Geometry: final body of the model. Coordinates: model frame, mm. A direction names the side the tool comes from. Round coordinates to 2 decimals unless told otherwise and drop trailing zeros. Write each loop counter-clockwise with the first axis right and the second up, starting at its lowest first coordinate (ties: lowest second). Pieces come first, ordered by that corner, then holes. Notation, with made-up numbers: (12.25, 48) - (71.25, 48) arc R28 ccw to (71.25, 76) - close; hole circle Ø9 at (76.25, -5.5). An arc over 180 degrees is marked (long way). Write each question's results on one line, items separated by ' | '.
Autodesk Inventor part; units mm, degrees
ref_plane "YZ Plane" through (0, 0, 0) normal (1, 0, 0) x (0, 1, 0)
ref_plane "XZ Plane" through (0, 0, 0) normal (0, 1, 0) x (-1, 0, 0)
ref_plane "XY Plane" through (0, 0, 0) normal (0, 0, 1) x (1, 0, 0)
sketch "Seal Outline" plane through (0, 0, 0) normal (0, 1, 0) x (-1, 0, 0)
  line L0 (-48, 41.5) -> (48, 41.5)
  line L1 (62, 34.9661) -> (62, -34.9661)
  line L2 (-62, -34.9661) -> (-62, 34.9661)
  line L3 (62, 41.5045) -> (62, 41.5)
  arc A0 (-49.8748, 41.9666) -> (-48, 41.5) centre (-48, 45.5) ccw
  arc A1 (48, 41.5) -> (49.8748, 41.9666) centre (48, 45.5) ccw
  line L4 (48, 41.5) -> (37.7809, 41.4967)
  line L5 (-49.8748, 41.9666) -> (-62, 34.9661)
  line L6 (49.8748, 41.9666) -> (62, 34.9661)
  line L7 (62, -41.5045) -> (62, -41.5)
  arc A2 (49.8748, -41.9666) -> (48, -41.5) centre (48, -45.5) ccw
  line L8 (48, -41.5) -> (37.7809, -41.4967)
  line L9 (-48, -41.5) -> (48, -41.5)
  arc A3 (-48, -41.5) -> (-49.8748, -41.9666) centre (-48, -45.5) ccw
  line L10 (-49.8748, -41.9666) -> (-62, -34.9661)
  line L11 (49.8748, -41.9666) -> (62, -34.9661)
  line L12 (-39, 38.5) -> (39, 38.5)
  line L13 (59, 18.5) -> (59, -18.5)
  line L14 (39, -38.5) -> (-39, -38.5)
  line L15 (-59, -18.5) -> (-59, 18.5)
  arc A4 (-59, -18.5) -> (-39, -38.5) centre (-39, -18.5) ccw
  arc A5 (-39, 38.5) -> (-59, 18.5) centre (-39, 18.5) ccw
  arc A6 (59, 18.5) -> (39, 38.5) centre (39, 18.5) ccw
  arc A7 (39, -38.5) -> (59, -18.5) centre (39, -18.5) ccw
  point P0 (0, 0)
  dimension "d6" = 124
  dimension "d7" = 96
  dimension "d14" = 83
  dimension "d15" = 4
  dimension "d16" = 4
  dimension "d17" = 4
  dimension "d18" = 4
  dimension "d19" = 60
  dimension "d20" = 120
  dimension "d21" = 89.982
  dimension "d22" = 89.982
  dimension "d23" = 90
  dimension "d24" = 0
  dimension "d25" = 122.5631
  dimension "d26" = 122.5631
  dimension "d27" = 62
  dimension "d28" = 62
  dimension "d29" = 61.2816
  dimension "d30" = 61.2816
  dimension "d31" = 41.4847
  dimension "d32" = 41.4847
  dimension "d33" = 41.5
  dimension "d34" = 5.6585
  dimension "d35" = 66.2216
  dimension "d36" = 24.2191
  dimension "d37" = 24.2191
  dimension "d38" = 110
  dimension "d39" = 78
  dimension "d40" = 20
  dimension "d41" = 37
  dimension "d43" = 3
  dimension "d44" = 3
extrude "Extrusion1" add sketch "Seal Outline" along normal blind 1.85
sketch "Sketch2" plane through (0, 0, 0) normal (0, -1, 0) x (1, 0, 0)
  line L0 (62, 34.9661) -> (62, -34.9661)
  line L1 (-48, 41.5) -> (48, 41.5)
  line L2 (-62, -34.9661) -> (-62, 34.9661)
  line L3 (-48, 41.5) -> (-46.9319, 43.35)
  line L4 (-46.9319, 43.35) -> (46.9319, 43.35)
  line L5 (46.9319, 43.35) -> (48, 41.5)
  line L6 (-62, 34.9661) -> (-63.85, 33.898)
  line L7 (-63.85, 33.898) -> (-63.85, -33.898)
  line L8 (-63.85, -33.898) -> (-62, -34.9661)
  line L9 (62, 34.9661) -> (63.85, 33.898)
  line L10 (63.85, 33.898) -> (63.85, -33.898)
  line L11 (63.85, -33.898) -> (62, -34.9661)
  point P0 (-48, -41.5)
  point P1 (48, -41.5)
  dimension "d47" = 120
  dimension "d49" = 120
  dimension "d50" = 1.85
  dimension "d51" = 120
  dimension "d55" = 120
  dimension "d57" = 1.85
  dimension "d58" = 120
  dimension "d59" = 120
  dimension "d60" = 1.85
extrude "Extrusion3" add sketch "Sketch2" against normal blind 5
equation "\"d49\" = d47"
equation "\"d51\" = d47"
equation "\"d55\" = d47"
equation "\"d57\" = d50"
equation "\"d58\" = d47"
equation "\"d59\" = d47"
equation "\"d60\" = d50"
properties part number "RubberLidSeal" material "Rubber"
Q1. Section query C-C, the plane z = -0.5. Return loops of the section in (x, y), plus the area to 3 significant figures.
Answer block:
outline: (-63.85, 0) - (-59, 0) - (-59, 1.85) - (-62, 1.85) - (-62, 5) - (-63.85, 5) - close; (59, 0) - (63.85, 0) - (63.85, 5) - (62, 5) - (62, 1.85) - (59, 1.85) - close | area: 29.6 mm2
Q2. Ray query, line 1 along Z through (x, y) = (-29, 0.85); line 2 along X through (y, z) = (4, 25.5); line 3 along X through (y, z) = (0.7, 13.5). Return the intervals inside material, ascending.
Answer block:
line 1: -41.5 to -38.5, 38.5 to 43.35 | line 2: -63.85 to -62, 62 to 63.85 | line 3: -63.85 to -59, 59 to 63.85
Q3. Pin query (flat end, axial travel): pin 1 (0.9 mm diameter, centred on x = -9.5, y = 0.5, fed in from -Z); pin 2 (3 mm diameter, centred on x = 11, y = 4, fed in from -Z). Return the tip coordinate at first contact, or that it passes through.
Answer block:
pin 1: z = -41.5 | pin 2: z = 41.5
Q4. Access query for faces 4 (the flat face through (5, 1.85, -40)), 5 (the flat face through (-1, 3, 41.5)), 6 (the cylindrical face through (52.986, 0.912, -32.797)). Directions: +Z, -Z, +X, -X, +Y, -Y. A direction counts if a zero-diameter tool reaches every point of the face in a straight line with its end or side. Return the directions, or none.
Answer block:
face 4: -Z, +Y | face 5: -Z, +X, -X, +Y | face 6: +Y, -Y
Q5. Section query B-B, the plane y = 3. Return loops of the section in (x, z), plus the area to 3 significant figures.
Answer block:
outline: (-63.85, -33.9) - (-62, -34.97) - (-62, 34.97) - (-63.85, 33.9) - close; (-48, 41.5) - (48, 41.5) - (46.93, 43.35) - (-46.93, 43.35) - close; (62, -34.97) - (63.85, -33.9) - (63.85, 33.9) - (62, 34.97) - close | area: 430 mm2
Q6. Section query D-D, the plane z = 28.5. Return loops of the section in (x, y).
Answer block:
outline: (-63.85, 0) - (-56.32, 0) - (-56.32, 1.85) - (-62, 1.85) - (-62, 5) - (-63.85, 5) - close; (56.32, 0) - (63.85, 0) - (63.85, 5) - (62, 5) - (62, 1.85) - (56.32, 1.85) - close
Q7. Mould query, pull axis X, two halves, no side actions, for faces 1 (the flat face through (-63.85, 2, 0)), 2 (the flat face through (63.85, 2, 0)), 3 (the cylindrical face through (-52.986, 0.912, 32.797)). Classes: pulls with the +X half, pulls with the -X half, needs draft (parallel to the pull), parting line crosses it, or undercut.
Answer block:
face 1: pulls with the -X half | face 2: pulls with the +X half | face 3: undercut
Q8. Section query A-A, the plane x = 17. Return loops of the section in (y, z).
Answer block:
outline: (0, -41.5) - (1.85, -41.5) - (1.85, -38.5) - (0, -38.5) - close; (0, 38.5) - (1.85, 38.5) - (1.85, 41.5) - (5, 41.5) - (5, 43.35) - (0, 43.35) - close
